Can you work these out from the model? Positions are in its coordinate system, mm. A direction names the side the tool comes from. Give positions to 0.01 mm unless a question says otherwise; leave off trailing zeros. Order: outer loops, then holes, each group sorted by start corner. A loop starts at its lowest first (then second) coordinate and runs counter-clockwise, first axis right, second up. Notation, with made-up numbers: (0.25, 85) - (6.25, 85) arc R17 ccw to (6.25, 102) - close; hole circle Ø6 at (19.5, 44). An arc over 180 degrees is marked (long way). Answer as a JSON object with one key per item and string values.
```python
from build123d import *

# Parameters (mm, degrees)
SKETCH1_W               = 22
SKETCH1_H               = 10
BOSS_EXTRUDE1_DEPTH     = 25
FILLET1_R               = 5
FILLET2_R               = 5
FILLET3_R               = 5
FILLET4_R               = 5
FILLET5_R               = 2
FILLET6_R               = 1
FILLET7_R               = 3
FILLET8_R               = 5
CUT_EXTRUDE1_DEPTH      = 35
CUT_EXTRUDE1_DEPTH_BACK = 25
SKETCH2_W               = 5.25
SKETCH2_H               = 2
BOSS_EXTRUDE2_DEPTH     = 25
FILLET9_R               = 1


# Some blends are built 0.0001 mm under size
with BuildPart() as part:
    # Sketch1 → Boss-Extrude1 (new body)
    with BuildSketch(Plane(origin=(0, 0, 0), x_dir=(0, 0, -1), z_dir=(1, 0, 0))):
        with BuildLine():
            ThreePointArc((-15.5, -17.5), (-60.5, -62.5), (-15.5, -107.5))
            Line((-15.5, -107.5), (19.5, -107.5))
            Line((19.5, -107.5), (19.5, -127.5))
            Line((19.5, -127.5), (-15.5, -127.5))
            ThreePointArc((-15.5, -127.5), (-80.4518339, -65.001853916), (-20.5, 2.307406984))
            Line((-20.5, 2.307406984), (-15.5, 32.5))
            Line((-15.5, 32.5), (-10.5, 32.5))
            Line((-10.5, 32.5), (-10.5, 2.5))
            Line((-10.5, 2.5), (10.5, 2.5))
            Line((10.5, 2.5), (10.5, 32.5))
            Line((10.5, 32.5), (15.5, 32.5))
            Line((15.5, 32.5), (20.8, -2.5))
            Line((20.8, -2.5), (0, -17.5))
            Line((0, -17.5), (-15.5, -17.5))
        make_face()
        with BuildLine():
            ThreePointArc((-55.647836382, -107.088689529), (-37.002076973, -118.51482559), (-15.5, -122.5))
            Line((-15.5, -122.5), (-15.5, -112.5))
            ThreePointArc((-15.5, -112.5), (-33.418397477, -109.179021325), (-48.956530318, -99.657241274))
            Line((-48.956530318, -99.657241274), (-55.647836382, -107.088689529))
        make_face(mode=Mode.SUBTRACT)
        with BuildLine():
            ThreePointArc((-60.088689529, -22.352163618), (-70.932771951, -39.538994058), (-75.417772085, -59.359842625))
            Line((-75.417772085, -59.359842625), (-65.431476738, -59.883202188))
            ThreePointArc((-65.431476738, -59.883202188), (-61.693976626, -43.365828382), (-52.657241274, -29.043469682))
            Line((-52.657241274, -29.043469682), (-60.088689529, -22.352163618))
        make_face(mode=Mode.SUBTRACT)
        with BuildLine():
            ThreePointArc((-21.771707796, -2.828686278), (-39.904198585, -7.687272541), (-55.647836382, -17.911310471))
            Line((-55.647836382, -17.911310471), (-48.956530318, -25.342758726))
            ThreePointArc((-48.956530318, -25.342758726), (-35.836832154, -16.822727118), (-20.726423163, -12.773905232))
            Line((-20.726423163, -12.773905232), (-21.771707796, -2.828686278))
        make_face(mode=Mode.SUBTRACT)
        Polygon((8.463652775, -2.5), (-7.917479229, -12.773905232), (-10.5, -12.773905232), (-10.5, -2.5), align=None, mode=Mode.SUBTRACT)
        with Locations((1.5, -117.5)):
            Rectangle(SKETCH1_W, SKETCH1_H, mode=Mode.SUBTRACT)
        with BuildLine():
            Line((-65.431476738, -65.116797812), (-75.417772085, -65.640157375))
            ThreePointArc((-75.417772085, -65.640157375), (-70.932771951, -85.461005942), (-60.088689529, -102.647836382))
            Line((-60.088689529, -102.647836382), (-52.657241274, -95.956530318))
            ThreePointArc((-52.657241274, -95.956530318), (-61.693976626, -81.634171618), (-65.431476738, -65.116797812))
        make_face(mode=Mode.SUBTRACT)
    extrude(amount=-BOSS_EXTRUDE1_DEPTH)

    # Fillet1
    fillet1_edges = [part.edges().sort_by_distance(p)[0] for p in [
        (-12.5, -99.657241274, 48.956530318),
        (-12.5, -112.5, 9.5),
        (-12.5, -122.5, 9.5),
        (-12.5, -122.5, 15.5),
        (-12.5, -122.5, -12.5),
        (-12.5, -112.5, -12.5),
        (-12.5, -107.088689529, 55.647836382),
        (-12.5, -112.5, 15.5),
        (-12.5, -95.956530318, 52.657241274),
        (-12.5, -102.647836382, 60.088689529),
        (-12.5, -22.352163618, 60.088689529),
        (-12.5, -29.043469682, 52.657241274),
        (-12.5, -59.883202188, 65.431476738),
        (-12.5, -59.359842625, 75.417772085),
        (-12.5, -17.911310471, 55.647836382),
        (-12.5, -25.342758726, 48.956530318),
        (-12.5, -12.773905232, 20.726423163),
        (-12.5, -2.828686278, 21.771707796),
    ]]
    fillet(fillet1_edges, radius=FILLET1_R - 0.0001)  # a hair under: the kernel refuses the full size

    # Fillet2
    fillet2_edges = [part.edges().sort_by_distance(p)[0] for p in [
        (-12.5, -65.116797812, 65.431476738),
        (-12.5, -65.640157375, 75.417772085),
    ]]
    fillet(fillet2_edges, radius=FILLET2_R - 0.0001)  # a hair under: the kernel refuses the full size

    # Fillet3
    fillet3_edges = [part.edges().sort_by_distance(p)[0] for p in [
        (-12.5, -2.5, 10.5),
    ]]
    fillet(fillet3_edges, radius=FILLET3_R)

    # Fillet4
    # the kernel refuses this fillet: 5 mm, written as the material it adds along each edge
    with BuildSketch(Plane(origin=(0, -12.773905232, 10.5), x_dir=(0, 1, 0), z_dir=(-1, 0, 0))) as fillet4_piece_1:
        with BuildLine():
            CenterArc((4.376733277, 5), FILLET4_R, 208.91397124, 61.08602876)
            Line((0, 2.582520771), (-0.087534666, 2.534171187))
            ThreePointArc((-0.087534666, 2.534171187), (-0.1, 1.291260386), (-0.1, 0))
            Line((-0.1, 0), (0, -0.1))
            Line((0, -0.1), (4.376733277, -0.1))
            Line((4.376733277, -0.1), (4.376733277, 0))
        make_face()
    extrude(amount=25)

    # Fillet5
    fillet5_edges = [part.edges().sort_by_distance(p)[0] for p in [
        (-12.5, -12.773905232, 7.917479229),
    ]]
    fillet(fillet5_edges, radius=FILLET5_R)

    # Fillet6
    fillet6_edges = [part.edges().sort_by_distance(p)[0] for p in [
        (-12.5, -2.5, -8.463652775),
    ]]
    fillet(fillet6_edges, radius=FILLET6_R)

    # Fillet7
    fillet7_edges = [part.edges().sort_by_distance(p)[0] for p in [
        (-12.5, 2.307406984, 20.5),
        (-12.5, -2.5, -20.8),
        (-12.5, -17.5, 0),
    ]]
    fillet(fillet7_edges, radius=FILLET7_R)

    # Fillet8
    fillet8_edges = [part.edges().sort_by_distance(p)[0] for p in [
        (-12.5, -107.5, -19.5),
        (-12.5, -127.5, -19.5),
    ]]
    fillet(fillet8_edges, radius=FILLET8_R)

    # Sketch2 → Cut-Extrude1 (cut, two sides: drawn at the far end of the back side and taken through both)
    with BuildSketch(Plane.XY.offset(-10.5).offset(-CUT_EXTRUDE1_DEPTH_BACK)):
        with Locations((-17.375, 24)):
            Rectangle(SKETCH2_W, SKETCH2_H)
        with Locations((-7.625, 24)):
            Rectangle(SKETCH2_W, SKETCH2_H)
    extrude(amount=CUT_EXTRUDE1_DEPTH + CUT_EXTRUDE1_DEPTH_BACK, mode=Mode.SUBTRACT)

    # Sketch3 → Boss-Extrude2 (add)
    with BuildSketch(Plane(origin=(0, 0, 0), x_dir=(0, 0, -1), z_dir=(1, 0, 0))):
        Polygon((16.635714286, 25), (18.635714286, 25.302857143), (15.5, 32.5), align=None)
        Polygon((-16.742026479, 25), (-18.742026479, 25.331207061), (-15.5, 32.5), align=None)
    extrude(amount=-BOSS_EXTRUDE2_DEPTH)

    # Fillet9
    fillet9_edges = [part.edges().sort_by_distance(p)[0] for p in [
        (-12.5, 25.302857143, -18.635714286),
        (-12.5, 25.331207061, 18.742026479),
    ]]
    fillet(fillet9_edges, radius=FILLET9_R)


solid = part.part
```
Q1. Which directions (+Z, -Z, +X, -X, +Y, -Y) give clear straight access to the entire face, cutting with the end or side of a thin tool? Please do faces 4 (the face through (-17, 23, 14)), 5 (the face through (-12.68, -3.93, 9)), 6 (the face through (-12.32, -10.16, -10.18)).
Recorded:
{"face 4": "+Z, -Z", "face 5": "+X, -X", "face 6": "-Z, +X, -X"}
Q2. If we section it at C-C, the plane x = -1.75: Count the separate pieces of the cut face and the enclosed holes in it, then the cut area to 3 significant figures.
Recorded:
{"separate pieces": "1", "enclosed holes": "6", "area": "3,460 mm^2"}
Q3. We'd pull the mould along Z, two halves only. Please class faces 1 (the face through (-12, -112.5, -1)), 2 (the face through (-8, 25, 14)), 3 (the face through (-12.325, 29.456, -16.826)): released by +Z, released by -Z, zero draft, split by the parting line, or undercut.
Recorded:
{"face 1": "undercut", "face 2": "zero draft", "face 3": "released by -Z"}
Q4. If we section it at A-A, the plane y = 12.5: Please give me the cut outline in (x, z).
Recorded:
{"outline": "(-25, -18.53) - (0, -18.53) - (0, -10.5) - (-25, -10.5) - close; (-25, 10.5) - (0, 10.5) - (0, 18.81) - (-25, 18.81) - close"}
Q5. If we section it at D-D, the plane y = -83.5: Please give me the cut outline in (x, z), then the cut area to 3 significant figures.
Recorded:
{"outline": "(-25, 55.3) - (0, 55.3) - (0, 60.88) - (-25, 60.88) - close; (-25, 71.7) - (0, 71.7) - (0, 77.01) - (-25, 77.01) - close", "area": "272 mm^2"}
Q6. If we section it at B-B, the plane z = 48: Please give me the cut outline in (x, y), then the cut area to 3 significant figures.
Recorded:
{"outline": "(-25, -118.79) - (0, -118.79) - (0, -112.94) - (-25, -112.94) - close; (-25, -101.57) - (0, -101.57) - (0, -93.62) - (-25, -93.62) - close; (-25, -31.38) - (0, -31.38) - (0, -23.43) - (-25, -23.43) - close; (-25, -12.06) - (0, -12.06) - (0, -6.21) - (-25, -6.21) - close", "area": "690 mm^2"}
Q7. I need wall thicknesses on L1, parallel to Z at x = -22.75, y = 20.5; L2, parallel to Y at x = -20.5, z = 16.5; L3, parallel to Y at x = -6.25, z = -12. Which ranges of each line are inside material? Lowest first, please.
Recorded:
{"L1": "z = -17.32 to -10.5, 10.5 to 17.49", "L2": "y = -127.49 to -120.27, -114.27 to -107.49, -17.51 to 30.29", "L3": "y = -127.5 to -119.68, -115.32 to -107.5, -8.85 to 23, 25 to 32.5"}
Q8. I'm going to push flat-ended pins straight in: pin 1 Ø2 at (x, y) = (-5.5, -93) entering from -Z; pin 2 Ø8 at (x, y) = (-15.5, -116) entering from -Z; pin 3 Ø0.6 at (y, z) = (24, 14.5) entering from +X; pin 4 Ø1.5 at (x, y) = (-19, -79) entering from -Z. Where does each tip first touch, or does it pass through?
Recorded:
{"pin 1": "stops at z = 47.64", "pin 2": "stops at z = -19.5", "pin 3": "stops at x = 0", "pin 4": "stops at z = 57.06"}
